```python
from build123d import *

# Parameters (mm, degrees)
IZIM1_R                     = 2.5
Y_KSEKLIK_EKSTR_ZYON1_DEPTH = 30


with BuildPart() as part:
    # Çizim1 → Yükseklik-Ekstrüzyon1 (new body)
    with BuildSketch(Plane.XY):
        with BuildLine():
            Line((8.6, 3.3), (8.6, 6.402943725))
            ThreePointArc((8.6, 6.402943725), (8.291341716, 6.864883491), (7.746446609, 6.756497116))
            Line((7.746446609, 6.756497116), (4.646446609, 3.656497116))
            ThreePointArc((4.646446609, 3.656497116), (4.538060234, 3.494285441), (4.5, 3.302943725))
            Line((4.5, 3.302943725), (4.5, 0))
            Line((4.5, 0), (4.5, -3.302943725))
            ThreePointArc((4.5, -3.302943725), (4.538060234, -3.494285441), (4.646446609, -3.656497116))
            Line((4.646446609, -3.656497116), (7.746446609, -6.756497116))
            ThreePointArc((7.746446609, -6.756497116), (8.291341716, -6.864883491), (8.6, -6.402943725))
            Line((8.6, -6.402943725), (8.6, -3.3))
            ThreePointArc((8.6, -3.3), (8.629289322, -3.229289322), (8.7, -3.2))
            Line((8.7, -3.2), (9.4, -3.2))
            ThreePointArc((9.4, -3.2), (9.470710678, -3.229289322), (9.5, -3.3))
            Line((9.5, -3.3), (9.5, -3.8))
            ThreePointArc((9.5, -3.8), (9.529289322, -3.870710678), (9.6, -3.9))
            Line((9.6, -3.9), (9.9, -3.9))
            ThreePointArc((9.9, -3.9), (9.970710678, -3.929289322), (10, -4))
            Line((10, -4), (10, -9.5))
            ThreePointArc((10, -9.5), (9.853553391, -9.853553391), (9.5, -10))
            Line((9.5, -10), (4, -10))
            ThreePointArc((4, -10), (3.929289322, -9.970710678), (3.9, -9.9))
            Line((3.9, -9.9), (3.9, -9.6))
            ThreePointArc((3.9, -9.6), (3.870710678, -9.529289322), (3.8, -9.5))
            Line((3.8, -9.5), (3.3, -9.5))
            ThreePointArc((3.3, -9.5), (3.229289322, -9.470710678), (3.2, -9.4))
            Line((3.2, -9.4), (3.2, -8.7))
            ThreePointArc((3.2, -8.7), (3.229289322, -8.629289322), (3.3, -8.6))
            Line((3.3, -8.6), (6.402943725, -8.6))
            ThreePointArc((6.402943725, -8.6), (6.864883491, -8.291341716), (6.756497116, -7.746446609))
            Line((6.756497116, -7.746446609), (3.656497116, -4.646446609))
            ThreePointArc((3.656497116, -4.646446609), (3.494285441, -4.538060234), (3.302943725, -4.5))
            Line((3.302943725, -4.5), (0, -4.5))
            Line((0, -4.5), (-3.302943725, -4.5))
            ThreePointArc((-3.302943725, -4.5), (-3.494285441, -4.538060234), (-3.656497116, -4.646446609))
            Line((-3.656497116, -4.646446609), (-6.756497116, -7.746446609))
            ThreePointArc((-6.756497116, -7.746446609), (-6.864883491, -8.291341716), (-6.402943725, -8.6))
            Line((-6.402943725, -8.6), (-3.3, -8.6))
            ThreePointArc((-3.3, -8.6), (-3.229289322, -8.629289322), (-3.2, -8.7))
            Line((-3.2, -8.7), (-3.2, -9.4))
            ThreePointArc((-3.2, -9.4), (-3.229289322, -9.470710678), (-3.3, -9.5))
            Line((-3.3, -9.5), (-3.8, -9.5))
            ThreePointArc((-3.8, -9.5), (-3.870710678, -9.529289322), (-3.9, -9.6))
            Line((-3.9, -9.6), (-3.9, -9.9))
            ThreePointArc((-3.9, -9.9), (-3.929289322, -9.970710678), (-4, -10))
            Line((-4, -10), (-9.5, -10))
            ThreePointArc((-9.5, -10), (-9.853553391, -9.853553391), (-10, -9.5))
            Line((-10, -9.5), (-10, -4))
            ThreePointArc((-10, -4), (-9.970710678, -3.929289322), (-9.9, -3.9))
            Line((-9.9, -3.9), (-9.6, -3.9))
            ThreePointArc((-9.6, -3.9), (-9.529289322, -3.870710678), (-9.5, -3.8))
            Line((-9.5, -3.8), (-9.5, -3.3))
            ThreePointArc((-9.5, -3.3), (-9.470710678, -3.229289322), (-9.4, -3.2))
            Line((-9.4, -3.2), (-8.7, -3.2))
            ThreePointArc((-8.7, -3.2), (-8.629289322, -3.229289322), (-8.6, -3.3))
            Line((-8.6, -3.3), (-8.6, -6.402943725))
            ThreePointArc((-8.6, -6.402943725), (-8.291341716, -6.864883491), (-7.746446609, -6.756497116))
            Line((-7.746446609, -6.756497116), (-4.646446609, -3.656497116))
            ThreePointArc((-4.646446609, -3.656497116), (-4.538060234, -3.494285441), (-4.5, -3.302943725))
            Line((-4.5, -3.302943725), (-4.5, 0))
            Line((-4.5, 0), (-4.5, 3.302943725))
            ThreePointArc((-4.5, 3.302943725), (-4.538060234, 3.494285441), (-4.646446609, 3.656497116))
            Line((-4.646446609, 3.656497116), (-7.746446609, 6.756497116))
            ThreePointArc((-7.746446609, 6.756497116), (-8.291341716, 6.864883491), (-8.6, 6.402943725))
            Line((-8.6, 6.402943725), (-8.6, 3.3))
            ThreePointArc((-8.6, 3.3), (-8.629289322, 3.229289322), (-8.7, 3.2))
            Line((-8.7, 3.2), (-9.4, 3.2))
            ThreePointArc((-9.4, 3.2), (-9.470710678, 3.229289322), (-9.5, 3.3))
            Line((-9.5, 3.3), (-9.5, 3.8))
            ThreePointArc((-9.5, 3.8), (-9.529289322, 3.870710678), (-9.6, 3.9))
            Line((-9.6, 3.9), (-9.9, 3.9))
            ThreePointArc((-9.9, 3.9), (-9.970710678, 3.929289322), (-10, 4))
            Line((-10, 4), (-10, 9.5))
            ThreePointArc((-10, 9.5), (-9.853553391, 9.853553391), (-9.5, 10))
            Line((-9.5, 10), (-4, 10))
            ThreePointArc((-4, 10), (-3.929289322, 9.970710678), (-3.9, 9.9))
            Line((-3.9, 9.9), (-3.9, 9.6))
            ThreePointArc((-3.9, 9.6), (-3.870710678, 9.529289322), (-3.8, 9.5))
            Line((-3.8, 9.5), (-3.3, 9.5))
            ThreePointArc((-3.3, 9.5), (-3.229289322, 9.470710678), (-3.2, 9.4))
            Line((-3.2, 9.4), (-3.2, 8.7))
            ThreePointArc((-3.2, 8.7), (-3.229289322, 8.629289322), (-3.3, 8.6))
            Line((-3.3, 8.6), (-6.402943725, 8.6))
            ThreePointArc((-6.402943725, 8.6), (-6.864883491, 8.291341716), (-6.756497116, 7.746446609))
            Line((-6.756497116, 7.746446609), (-3.656497116, 4.646446609))
            ThreePointArc((-3.656497116, 4.646446609), (-3.494285441, 4.538060234), (-3.302943725, 4.5))
            Line((-3.302943725, 4.5), (0, 4.5))
            Line((0, 4.5), (3.302943725, 4.5))
            ThreePointArc((3.302943725, 4.5), (3.494285441, 4.538060234), (3.656497116, 4.646446609))
            Line((3.656497116, 4.646446609), (6.756497116, 7.746446609))
            ThreePointArc((6.756497116, 7.746446609), (6.864883491, 8.291341716), (6.402943725, 8.6))
            Line((6.402943725, 8.6), (3.3, 8.6))
            ThreePointArc((3.3, 8.6), (3.229289322, 8.629289322), (3.2, 8.7))
            Line((3.2, 8.7), (3.2, 9.4))
            ThreePointArc((3.2, 9.4), (3.229289322, 9.470710678), (3.3, 9.5))
            Line((3.3, 9.5), (3.8, 9.5))
            ThreePointArc((3.8, 9.5), (3.870710678, 9.529289322), (3.9, 9.6))
            Line((3.9, 9.6), (3.9, 9.9))
            ThreePointArc((3.9, 9.9), (3.929289322, 9.970710678), (4, 10))
            Line((4, 10), (9.5, 10))
            ThreePointArc((9.5, 10), (9.853553391, 9.853553391), (10, 9.5))
            Line((10, 9.5), (10, 4))
            ThreePointArc((10, 4), (9.970710678, 3.929289322), (9.9, 3.9))
            Line((9.9, 3.9), (9.6, 3.9))
            ThreePointArc((9.6, 3.9), (9.529289322, 3.870710678), (9.5, 3.8))
            Line((9.5, 3.8), (9.5, 3.3))
            ThreePointArc((9.5, 3.3), (9.470710678, 3.229289322), (9.4, 3.2))
            Line((9.4, 3.2), (8.7, 3.2))
            ThreePointArc((8.7, 3.2), (8.629289322, 3.229289322), (8.6, 3.3))
        make_face()
        Circle(IZIM1_R, mode=Mode.SUBTRACT)
    extrude(amount=Y_KSEKLIK_EKSTR_ZYON1_DEPTH)


solid = part.part
```
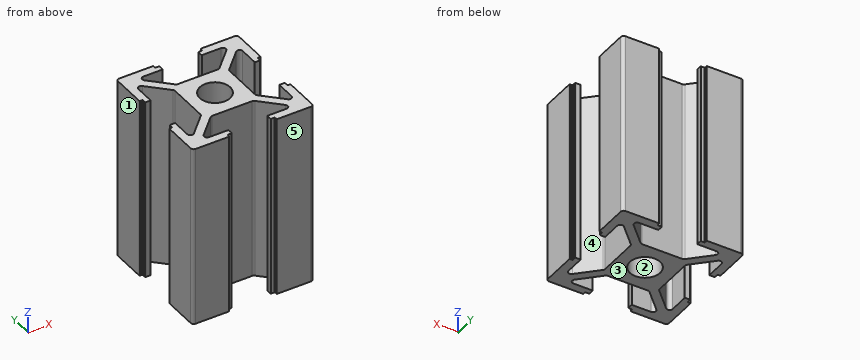
The model under review builds one solid part; all positions refer to its coordinate system, in mm. Face numbers are marked on the shaded views. A direction names the side the tool comes from. Give positions to 0.01 mm unless a question says otherwise; leave off trailing zeros. Write each loop counter-clockwise with the first axis right and the second up, starting at its lowest first coordinate (ties: lowest second). Pieces come first, ordered by that corner, then holes. Notation, with made-up numbers: M 69,27.5 L 77,27.5 A17 cw 77,53.5 Z; hole C -29.5,32 d10. An arc over 180 degrees is marked long. Write item = value, one per line. Start each with the question number.
Q1. We need section A-A (x = 0). State the section outline as (y, z) points.
Q2. Machinability: for the marked faces 4 and 5, which of the approach directions +Z, -Z, +X, -X, +Y, -Y give a long, thin tool a straight path to every point of the face, cutting with its end or side? Answer none if there is none.
Q3. For line 1 (Y direction, x = 0, z = 7.5); line 2 (Y direction, x = 5.25, z = 15.25), list the stretches that pass through material, from the lowest coordinate up.
Q4. We need section C-C (y = -5). State the section outline as (x, z) points, plus the area to 3 significant figures.
Q5. Clearance check with flat-ended pins moving along their axes: pin 1 (3 mm diameter, centred on x = 0.5, z = 15, fed in from +Y); pin 2 (0.6 mm diameter, centred on x = -3.5, z = 8.5, fed in from +Y). State where each tip first meets the part, or that it passes through.
Q6. Mouldability with a two-part tool opening along X and no side actions: class the marked faces 1, 2 and 3 as released by +X, released by -X, zero draft, split by the parting line, or undercut.
Result set:
q1.outline = M -4.5,0 L -2.5,0 L -2.5,30 L -4.5,30 Z; M 2.5,0 L 4.5,0 L 4.5,30 L 2.5,30 Z
q2.face_4 = +Z, -Z
q2.face_5 = +Z, -Z, +X, -X, -Y
q3.line_1 = -4.5 to -2.5, 2.5 to 4.5
q3.line_2 = -10 to -8.6, -6.24 to -4.26, 4.26 to 6.24, 8.6 to 10
q4.outline = M -10,0 L -8.6,0 L -8.6,30 L -10,30 Z; M -5.99,0 L -4.01,0 L -4.01,30 L -5.99,30 Z; M 4.01,0 L 5.99,0 L 5.99,30 L 4.01,30 Z; M 8.6,0 L 10,0 L 10,30 L 8.6,30 Z
q4.area = 203 mm2
q5.pin_1 = 4.5
q5.pin_2 = 9.5
q6.face_1 = released by -X
q6.face_2 = undercut
q6.face_3 = zero draft
